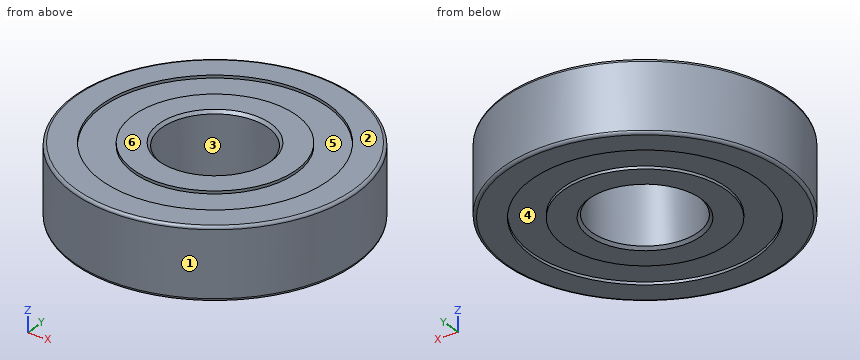
Autodesk Inventor part; units mm, degrees
ref_plane "Work Plane1" through (0, 0, 1.5875) normal (0, 0, 1) x (1, 0, 0)
ref_plane "YZ Plane" through (0, 0, 0) normal (1, 0, 0) x (0, 1, 0)
ref_plane "XZ Plane" through (0, 0, 0) normal (0, 1, 0) x (-1, 0, 0)
sketch "Sketch1" plane through (0, 0, 0) normal (0, 0, 1) x (1, 0, 0)
  circle A0 centre (0, 0) radius 2.3813
  circle A1 centre (0, 0) radius 6.35
  circle A2 centre (0, 0) radius 3.6512
  circle A3 centre (0, 0) radius 5.08
  dimension "d0" = 4.7625
  dimension "d1" = 12.7
  dimension "d2" = 1.27
  dimension "d3" = 1.27
extrude "Extrusion1" add sketch "Sketch1" along normal blind 3.175
fillet "Fillet1" radius 0.127 2 edges at (-6.35, 0, 3.175) (-6.35, 0, 0)
chamfer "Chamfer1" distance 0.127 angle 45 2 edges at (-2.3813, 0, 3.175) (-2.3813, 0, 0)
ref_plane "Work Plane1" through (0, 0, 1.5875) normal (0, 0, 1) x (1, 0, 0)
sketch "Sketch2" plane through (0, 0, 1.5875) normal (0, 0, 1) x (1, 0, 0)
  circle A0 centre (0, 0) radius 2.3813
  circle A1 centre (0, 0) radius 3.6512
  circle A2 centre (0, 0) radius 6.35
  circle A3 centre (0, 0) radius 5.08
extrude "Extrusion2" add sketch "Sketch2" along normal mid plane 2.921 contours A3
properties part number "Rear Hub Bearing"
Input: part model. Units: mm. Frame: model coordinates. Face numbers are marked on the shaded views. A direction names the side the tool comes from. Coordinates: 2 decimals unless noted, no trailing zeros. Use a Markdown table: item, result. Add a question column.
1) Set-up query: the marked faces 4, 5 and 6. Return all of +Z, -Z, +X, -X, +Y, -Y with unobstructed straight access to the full face (end or side cutting, diameter ignored); none if empty.
2) Line query: L1, parallel to Y at x = 0, z = 3.1; L2, parallel to Y at x = 0, z = 1.4; L3, parallel to Z at x = 4, y = 2.5. Output: solid intervals per line, ascending. Write a range as from..to.
3) Pin query (flat end, axial travel): P1, Ø1.5, axis at y = -2.5, z = 0.5, coming from the -X side; P2, Ø1, axis at y = -3, z = 2, coming from the -X side. Return the tip coordinate at first contact, or that it passes through.
4) Draft query along X for the marked faces 1, 2 and 3. Return one class per face: +X half, -X half, draft (parallel to the pull), parting line (faces both ways), or undercut.
Answer below:
| question | item | result |
|---|---|---|
| 1 | face 4 | -Z |
| 1 | face 5 | +Z |
| 1 | face 6 | +Z, +X, -X, +Y, -Y |
| 2 | L1 | -6.34..-5.08, -3.65..-2.43, 2.43..3.65, 5.08..6.34 |
| 2 | L2 | -6.35..-2.38, 2.38..6.35 |
| 2 | L3 | 0.13..3.05 |
| 3 | P1 | x = -6.1 |
| 3 | P2 | x = -5.84 |
| 4 | face 1 | parting line |
| 4 | face 2 | draft |
| 4 | face 3 | undercut |
